The model under review builds one solid part; all positions refer to its coordinate system, in mm. A direction names the side the tool comes from. Coordinates: 2 decimals unless noted, no trailing zeros. Order: outer loops, then holes, each group sorted by start corner. A loop starts at its lowest first (then second) coordinate and runs counter-clockwise, first axis right, second up. Notation, with made-up numbers: M 7,-20.5 L 45,-20.5 A20 cw 45,0.5 Z; hole C 58.5,-29 d2. An arc over 180 degrees is marked long. Answer in a Markdown table with one row per item.
from build123d import *

# Parameters (mm, degrees)
EXTRUDE_THIN1_DEPTH      = 9.525
EXTRUDE_THIN1_DEPTH_BACK = 9.525


with BuildPart() as part:
    # Sketch1 → Extrude-Thin1 (new body, two sides)
    with BuildSketch(Plane.XY) as extrude_thin1_sk:
        with BuildLine():
            Line((264.851021428, -59.353801417), (-3.190403177, -24.621386578))
            ThreePointArc((-3.190403177, -24.621386578), (-24.82723, 0), (-3.190403177, 24.621386578))
            Line((-3.190403177, 24.621386578), (264.851021428, 59.353801417))
            ThreePointArc((264.851021428, 59.353801417), (332.39202, 0), (264.851021428, -59.353801417))
        make_face()
        with BuildLine():
            Line((265.17742208, -56.834860644), (-2.864002524, -22.102445806))
            ThreePointArc((-2.864002524, -22.102445806), (-22.28723, 0), (-2.864002524, 22.102445806))
            Line((-2.864002524, 22.102445806), (265.17742208, 56.834860644))
            ThreePointArc((265.17742208, 56.834860644), (329.85202, 0), (265.17742208, -56.834860644))
        make_face(mode=Mode.SUBTRACT)
    extrude(amount=EXTRUDE_THIN1_DEPTH)
    extrude(extrude_thin1_sk.sketch, amount=-EXTRUDE_THIN1_DEPTH_BACK)


solid = part.part
(1) Machinability: for faces 1 (the cylindrical face through (329.836, 1.364, 0.133)), 2 (the cylindrical face through (-24.822, -0.501, 0.133)), which of the approach directions +Z, -Z, +X, -X, +Y, -Y give a long, thin tool a straight path to every point of the face, cutting with its end or side? Answer none if there is none.
Report:
| item | result |
|---|---|
| face 1 | +Z, -Z |
| face 2 | +Z, -Z, -X |
(2) Take a section at A-A (y = 0). Write out the cut boundary in (x, z) (3 decimals), then the cut area to 3 significant figures.
Report:
| item | result |
|---|---|
| outline | M -24.827,-9.525 L -22.287,-9.525 L -22.287,9.525 L -24.827,9.525 Z; M 329.852,-9.525 L 332.392,-9.525 L 332.392,9.525 L 329.852,9.525 Z |
| area | 96.8 mm^2 |
(3) To check wall thickness, follow line 1 (Y direction, x = 277, z = 8); line 2 (Y direction, x = 158.5, z = -4.5); line 3 (X direction, y = -6, z = 4.5). State the ranges of each line that lie inside material, in increasing order. Write a range as [from, to].
Report:
| item | result |
|---|---|
| line 1 | [-59.68, -57.14], [57.14, 59.68] |
| line 2 | [-45.57, -43.01], [43.01, 45.57] |
| line 3 | [-24.09, -21.46], [329.54, 332.09] |
(4) Insertion check: P1, Ø4, axis at x = 142.5, z = -3, coming from the +Y side; P2, Ø1, axis at y = 14.5, z = -2, coming from the +X side; P3, Ø1.5, axis at x = 51.5, y = 27, coming from the +Z side; P4, Ø2, axis at y = -44, z = -2.5, coming from the +X side. Each pin has a flat end and moves straight along its axis. Give the tip position at first contact, or say it passes through.
Report:
| item | result |
|---|---|
| P1 | y = 43.76 |
| P2 | x = 330.73 |
| P3 | through |
| P4 | x = 314.17 |
(5) Take a section at C-C (x = 95.5). Write out the cut boundary in (y, z) (3 decimals), then the cut area to 3 significant figures.
Report:
| item | result |
|---|---|
| outline | M -37.41,-9.525 L -34.848,-9.525 L -34.848,9.525 L -37.41,9.525 Z; M 34.848,-9.525 L 37.41,-9.525 L 37.41,9.525 L 34.848,9.525 Z |
| area | 97.6 mm^2 |
(6) The part is to be moulded in two halves that separate along X. For faces 3 (the flat face through (128.954, 41.744, 0.133)), 4 (the cylindrical face through (-22.283, -0.45, 0.133)), 5 (the flat face through (155, -44, 9.525)), 6 (the flat face through (129.28, 39.226, 0.133)), say which applies: +X half, -X half, draft (parallel to the pull), parting line (faces both ways), or undercut.
Report:
| item | result |
|---|---|
| face 3 | -X half |
| face 4 | undercut |
| face 5 | draft |
| face 6 | undercut |
(7) Take a section at B-B (z = -6.5). Write out the cut boundary in (x, y), then the cut area to 3 significant figures.
Report:
| item | result |
|---|---|
| outline | M -3.19,-24.62 L 264.85,-59.35 A59.85 ccw long 264.85,59.35 L -3.19,24.62 A24.83 ccw Z; hole M -2.86,-22.1 L 265.18,-56.83 A57.31 ccw long 265.18,56.83 L -2.86,22.1 A22.29 ccw Z |
| area | 2,050 mm^2 |
